For this review, use the dimensioned drawing (mm, ordinates from the lowest corner) and the shaded views. Round coordinates to 2 decimals unless told otherwise and drop trailing zeros. Loops run counter-clockwise (first coordinate to the right, second up) from the corner with the lowest first, then second, coordinate; pieces in that order, holes last. Notation, with made-up numbers: (-0.5, 72.25) - (31.5, 72.25) arc R13 ccw to (31.5, 82.25) - close; hole circle Ø10 at (31.25, -22). An arc over 180 degrees is marked (long way). Use one line per item in the form item = value. Start each with the question number.
(1) We need section A-A, the plane y = 8. Write out the cut boundary in (x, z), then the cut area to 3 significant figures.
(2) We need section D-D, the plane y = 20.5. Write out the cut boundary in (x, z).
(3) For pin 1 (10 mm diameter, centred on y = 17, z = 7, fed in from -X); pin 2 (10 mm diameter, centred on y = 17.5, z = 8.5, fed in from -X); pin 3 (4 mm diameter, centred on x = 38, z = 35.5, fed in from +Y), all flat-tipped, find the tip position at first contact; note any pin that passes through.
(4) We need section C-C, the plane z = 6. Write out the cut boundary in (x, y), then the cut area to 3 significant figures.
(5) The part is to be moulded in two halves that separate along Y. For the marked faces 1, 2 and 3, say which applies: released by +Y, released by -Y, zero draft, split by the parting line, or undercut.
(6) Wall thickness on probe 1 along X at (y, z) = (25, 5); probe 2 along X at (y, z) = (25, 32): over which ranges is each line inside the solid? List them lowest first. Write a range as [from, to].
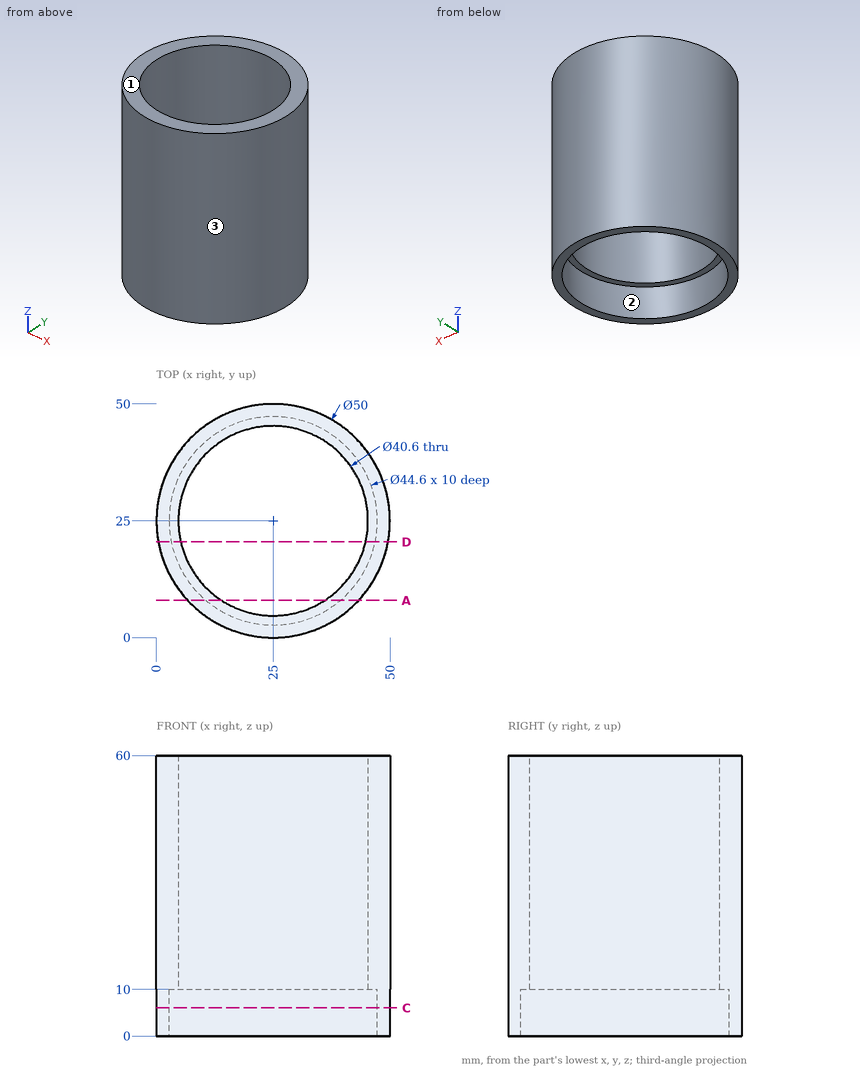
Data:
q1.outline = (6.67, 0) - (10.57, 0) - (10.57, 10) - (13.91, 10) - (13.91, 60) - (6.67, 60) - close; (36.09, 10) - (39.43, 10) - (39.43, 0) - (43.33, 0) - (43.33, 60) - (36.09, 60) - close
q1.area = 802 mm^2
q2.outline = (0.41, 0) - (3.16, 0) - (3.16, 10) - (5.21, 10) - (5.21, 60) - (0.41, 60) - close; (44.79, 10) - (46.84, 10) - (46.84, 0) - (49.59, 0) - (49.59, 60) - (44.79, 60) - close
q3.pin_1 = 0.18
q3.pin_2 = 0.13
q3.pin_3 = 47.45
q4.outline = circle Ø50 at (25, 25); hole circle Ø44.6 at (25, 25)
q4.area = 401 mm^2
q5.face_1 = zero draft
q5.face_2 = undercut
q5.face_3 = split by the parting line
q6.probe_1 = [0, 2.7], [47.3, 50]
q6.probe_2 = [0, 4.7], [45.3, 50]
